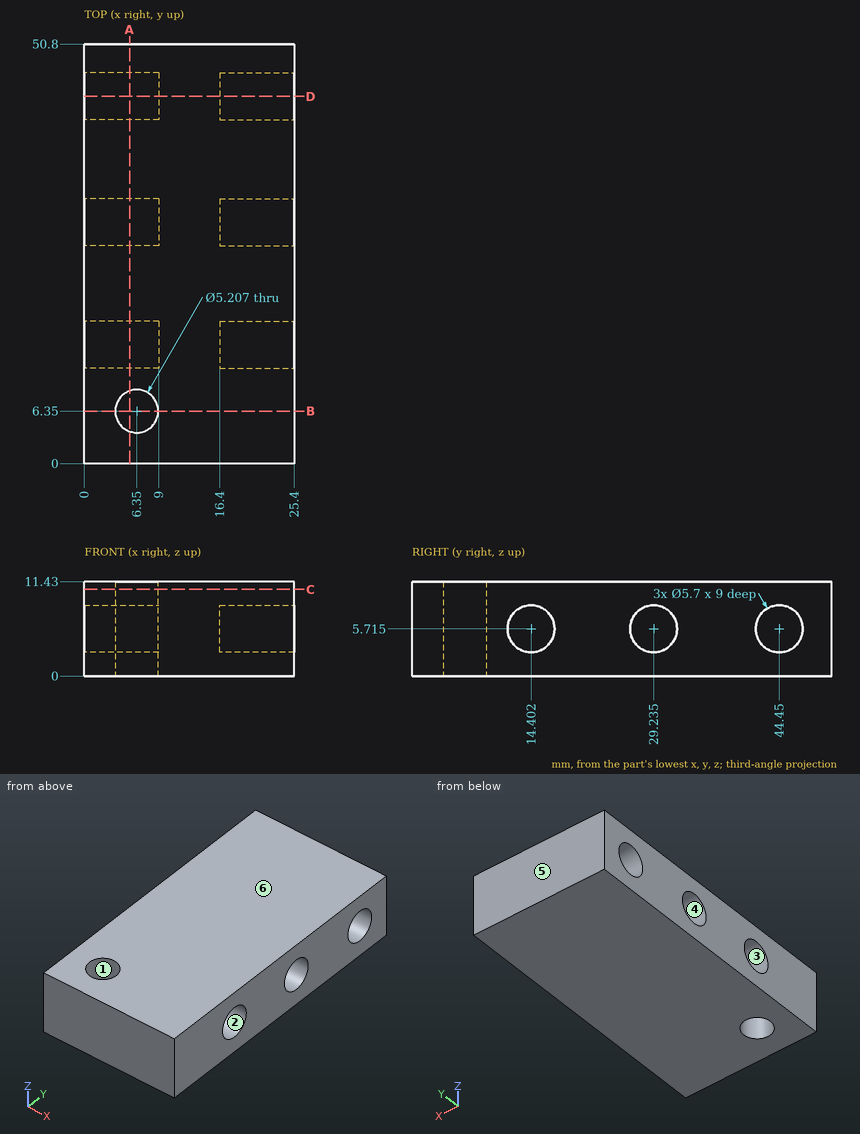
Design review of the part shown in the three views and the two pictorial views. Dimensions are in mm from the part's minimum x, y and z. A direction names the side the tool comes from. Coordinates: 2 decimals unless noted, no trailing zeros. Loops run counter-clockwise (first coordinate to the right, second up) from the corner with the lowest first, then second, coordinate; pieces in that order, holes last.
Q1. Tool access review of the marked faces 1, 2 and 3: name each direction out of +Z, -Z, +X, -X, +Y, -Y from which nothing blocks a thin tool from reaching the whole face with its end or side.
Reported:
face 1: +Z, -Z
face 2: +X
face 3: -X
Q2. The part is to be moulded in two halves that separate along Y. For the marked faces 4, 5 and 6, say which applies: +Y half, -Y half, draft (parallel to the pull), parting line (faces both ways), or undercut.
Reported:
face 4: undercut
face 5: +Y half
face 6: draft
Q3. We need section D-D on y = 44.45. State the section outline as (x, z) points (1 decimal), and give its area (3 significant figures).
Reported:
outline: (0, 0) - (25.4, 0) - (25.4, 2.9) - (16.4, 2.9) - (16.4, 8.6) - (25.4, 8.6) - (25.4, 11.4) - (0, 11.4) - (0, 8.6) - (9, 8.6) - (9, 2.9) - (0, 2.9) - close
area: 188 mm2
Q4. For pin 1 (1.7 mm diameter, centred on y = 29.5, z = 7, fed in from -X); pin 2 (3 mm diameter, centred on y = 32, z = 6, fed in from -X); pin 3 (1.7 mm diameter, centred on y = 29, z = 4.5, fed in from +X); pin 4 (3 mm diameter, centred on x = 6.35, y = 6.35, fed in from +Z), all flat-tipped, find the tip position at first contact; note any pin that passes through.
Reported:
pin 1: stops at x = 9
pin 2: stops at x = 0
pin 3: stops at x = 16.4
pin 4: passes through
Q5. We need section A-A on x = 5.5. State how many separate pieces and enclosed holes the cut face has, and give its area (3 significant figures).
Reported:
separate pieces: 2
enclosed holes: 3
area: 448 mm2
Q6. We need section B-B on y = 6.35. State the section outline as (x, z) points, and give its area (3 significant figures).
Reported:
outline: (0, 0) - (3.75, 0) - (3.75, 11.43) - (0, 11.43) - close; (8.95, 0) - (25.4, 0) - (25.4, 11.43) - (8.95, 11.43) - close
area: 231 mm2
Q7. We need section C-C on z = 10.5. State the section outline as (x, y) points, and give its area (3 significant figures).
Reported:
outline: (0, 0) - (25.4, 0) - (25.4, 50.8) - (0, 50.8) - close; hole circle Ø5.21 at (6.35, 6.35)
area: 1,270 mm2
Q8. To check wall thickness, follow line 1 (Y direction, x = 4.75, z = 7) (1 decimal); line 2 (Z direction, x = 22.75, y = 29.5); line 3 (Y direction, x = 22.5, z = 5) (1 decimal). State the ranges of each line that lie inside material, in increasing order.
Reported:
line 1: y = 0 to 4.3, 8.4 to 11.9, 16.9 to 26.7, 31.8 to 41.9, 47 to 50.8
line 2: z = 0 to 2.88, 8.55 to 11.43
line 3: y = 0 to 11.6, 17.2 to 26.5, 32 to 41.7, 47.2 to 50.8
